```python
from build123d import *

# Parameters (mm, degrees)
SKETCH_1_R          = 12
SKETCH_1_R_2        = 8
EXTRUDE_1_DEPTH     = 7.5
SKETCH_2_R          = 12
EXTRUDE_2_DEPTH     = 28
CUT_EXTRUDE_3_DEPTH = 11
SKETCH_4_R          = 7
CUT_EXTRUDE_4_DEPTH = 16
SKETCH_5_R          = 1.5
CUT_EXTRUDE_5_DEPTH = 30


with BuildPart() as part:
    # Эскиз1 → Вытянуть1 (new body)
    with BuildSketch(Plane(origin=(0, 0, 0), x_dir=(1, 0, 0), z_dir=(0, 1, 0))):
        with Locations(Location((0, 0, 0), (0, 0, 270))):
            Circle(SKETCH_1_R)
        with Locations(Location((0, 0, 0), (0, 0, 270))):
            Circle(SKETCH_1_R_2, mode=Mode.SUBTRACT)
    extrude(amount=EXTRUDE_1_DEPTH)

    # Эскиз2 → Вытянуть2 (add)
    with BuildSketch(Plane(origin=(0, 7.5, 0), x_dir=(1, 0, 0), z_dir=(0, 1, 0))):
        with Locations(Location((0, 0, 0), (0, 0, 270))):
            Circle(SKETCH_2_R)
    extrude(amount=EXTRUDE_2_DEPTH)

    # Эскиз3 → Вытянуть3 (cut)
    with BuildSketch(Plane.XZ.offset(-7.5)):
        Polygon((4.675379912, 1.625060824), (-1.625060824, 4.675379912), (-4.675379912, -1.625060824), (1.625060824, -4.675379912), align=None)
    extrude(amount=-CUT_EXTRUDE_3_DEPTH, mode=Mode.SUBTRACT)

    # Эскиз4 → Вытянуть4 (cut)
    with BuildSketch(Plane(origin=(0, 35.5, 0), x_dir=(1, 0, 0), z_dir=(0, 1, 0))):
        with Locations(Location((0, 0, 0), (0, 0, 270))):
            Circle(SKETCH_4_R)
    extrude(amount=-CUT_EXTRUDE_4_DEPTH, mode=Mode.SUBTRACT)

    # Эскиз5 → Вытянуть5 (cut, symmetric)
    with BuildSketch(Plane(origin=(0, 0, 0), x_dir=(0, 0, -1), z_dir=(1, 0, 0))):
        with Locations((0, 28.831403322)):
            Circle(SKETCH_5_R)
    extrude(amount=CUT_EXTRUDE_5_DEPTH, both=True, mode=Mode.SUBTRACT)


solid = part.part
```
CAD build for the part. Positions are in the model's coordinates, mm. A direction names the side the tool comes from. Coordinates: 2 decimals unless noted, no trailing zeros. Order: outer loops, then holes, each group sorted by start corner. A loop starts at its lowest first (then second) coordinate and runs counter-clockwise, first axis right, second up. Notation, with made-up numbers: (18, -36) - (39, -36) arc R31 cw to (39, 0) - close; hole circle Ø1 at (-6, 20.5). An arc over 180 degrees is marked (long way). Use a Markdown table: item, result. Add a question column.
(1) Flat gauge pins, fed straight in: pin 1 (4 mm diameter, centred on y = 28.5, z = -6.5, fed in from +X); pin 2 (12.5 mm diameter, centred on x = 0, z = 0, fed in from -Y); pin 3 (6 mm diameter, centred on x = 7, y = 16, fed in from -Z); pin 4 (1.8 mm diameter, centred on y = 28.83, z = 0, fed in from -X). Where does each tip first touch, or does it go through?
(2) Saw through at A-A (z = 0). Give the cut face in (x, y), then the cut area to 3 significant figures.
(3) Which spindle directions (+Z, -Z, +X, -X, +Y, -Y) get a long thin tool onto all of the face, cutting with end or side? Do faces 4 (the face through (0, 18.5, 0)), 5 (the face through (-5.2, 35.5, 5.2)), 6 (the face through (-6.21, 27.61, 3.23)). Say none if no direction does.
(4) Pull direction X, two halves, no side cores. Call faces 1 (the face through (-2, 0, 8)), 2 (the face through (1.57, 12.92, 3.13)), 3 (the face through (3.604, 17.502, 11.446)): +X half, -X half, draft (parallel to the pull), parting line (faces both ways), or undercut.
(5) Drill centre lines: line 1 along X through (y, z) = (4.75, 0); line 2 along X through (y, z) = (25.75, 0); line 3 along Y through (x, z) = (8.4, 0). Where is each one in solid material? Low to high. Write a range as [from, to].
(6) Saw through at D-D (x = -5.75). Give the cut face in (y, z).
(7) Saw through at B-B (x = 7.5). Give the cut face in (y, z).
(8) Saw through at C-C (y = 4.5). Give the cut face in (x, z), then the cut area to 3 significant figures.
Solved:
| question | item | result |
|---|---|---|
| 1 | pin 1 | stops at x = 11.12 |
| 1 | pin 2 | stops at y = 7.5 |
| 1 | pin 3 | stops at z = -11.31 |
| 1 | pin 4 | passes through |
| 2 | outline | (-12, 0) - (-8, 0) - (-8, 7.5) - (-3.89, 7.5) - (-3.89, 18.5) - (3.89, 18.5) - (3.89, 7.5) - (8, 7.5) - (8, 0) - (12, 0) - (12, 27.33) - (7, 27.33) - (7, 19.5) - (-7, 19.5) - (-7, 27.33) - (-12, 27.33) - close; (-12, 30.33) - (-7, 30.33) - (-7, 35.5) - (-12, 35.5) - close; (7, 30.33) - (12, 30.33) - (12, 35.5) - (7, 35.5) - close |
| 2 | area | 392 mm² |
| 3 | face 4 | -Y |
| 3 | face 5 | +Z, -Z, +X, -X, +Y |
| 3 | face 6 | +Y |
| 4 | face 1 | draft |
| 4 | face 2 | undercut |
| 4 | face 3 | parting line |
| 5 | line 1 | x = [-12, -8], [8, 12] |
| 5 | line 2 | x = [-12, -7], [7, 12] |
| 5 | line 3 | y = [0, 27.33], [30.33, 35.5] |
| 6 | outline | (0, -10.53) - (35.5, -10.53) - (35.5, -3.99) - (19.5, -3.99) - (19.5, 3.99) - (35.5, 3.99) - (35.5, 10.53) - (0, 10.53) - (0, 5.56) - (7.5, 5.56) - (7.5, -5.56) - (0, -5.56) - close |
| 7 | outline | (0, -9.37) - (35.5, -9.37) - (35.5, 9.37) - (0, 9.37) - (0, 2.78) - (7.5, 2.78) - (7.5, -2.78) - (0, -2.78) - close; hole circle Ø3 at (28.83, 0) |
| 8 | outline | circle Ø24 at (0, 0); hole circle Ø16 at (0, 0) |
| 8 | area | 251 mm² |
